For this review, use the dimensioned drawing (mm, ordinates from the lowest corner) and the shaded views. Coordinates: 2 decimals unless noted, no trailing zeros. Order: outer loops, then holes, each group sorted by start corner. A loop starts at its lowest first (then second) coordinate and runs counter-clockwise, first axis right, second up. Notation, with made-up numbers: (38, 89) -> (61, 89) arc R24 cw to (61, 103) -> close; hole circle Ø10 at (60, 37). An arc over 180 degrees is marked (long way). Return JSON: item names as keys, results as strings. Group by question number.
Item 1: Take a section at B-B (x = 43.1). Write out the cut boundary in (y, z), then the cut area to 3 significant figures.
Item 2: Take a section at A-A (z = 35.8). Write out the cut boundary in (x, y).
Item 3: Take a section at D-D (y = 2.15). Write out the cut boundary in (x, z).
Item 4: For line 1 along X through (y, z) = (2.3, 119.51); line 2 along X through (y, z) = (1.55, 5); line 3 along Z through (x, y) = (81, 1.35), list the stretches that pass through material, from the lowest coordinate up.
Item 5: Insertion check: pin 1 (1.5 mm diameter, centred on y = 2, z = 72.5, fed in from -X); pin 2 (0.9 mm diameter, centred on y = 1.5, z = 4.5, fed in from +X). Each pin has a flat end and moves straight along its axis. Give the tip position at first contact, or say it passes through.
Item 6: Take a section at C-C (z = 119.51). Write out the cut boundary in (x, y).
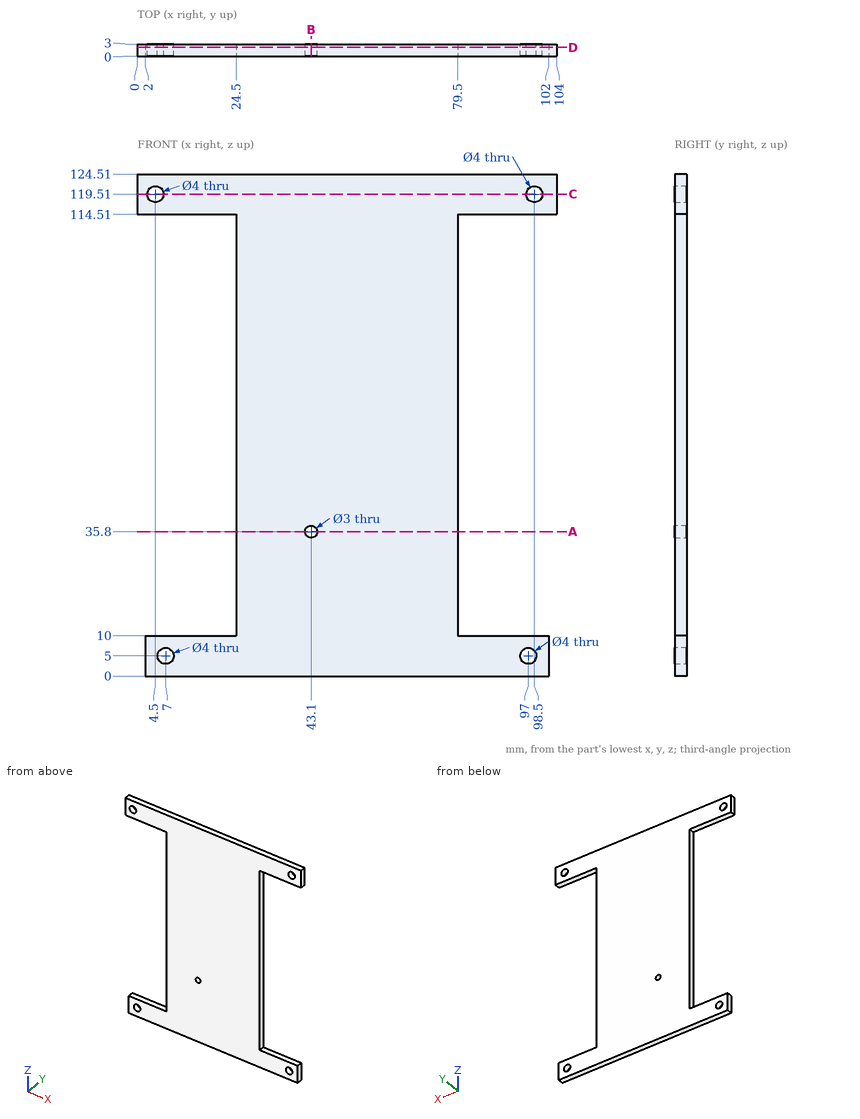
Findings below:
{
 "1": {"outline": "(0, 0) -> (3, 0) -> (3, 34.3) -> (0, 34.3) -> close; (0, 37.3) -> (3, 37.3) -> (3, 124.51) -> (0, 124.51) -> close", "area": "365 mm2"},
 "2": {"outline": "(24.5, 0) -> (41.6, 0) -> (41.6, 3) -> (24.5, 3) -> close; (44.6, 0) -> (79.5, 0) -> (79.5, 3) -> (44.6, 3) -> close"},
 "3": {"outline": "(0, 114.51) -> (24.5, 114.51) -> (24.5, 10) -> (2, 10) -> (2, 0) -> (102, 0) -> (102, 10) -> (79.5, 10) -> (79.5, 114.51) -> (104, 114.51) -> (104, 124.51) -> (0, 124.51) -> close; hole circle Ø4 at (4.5, 119.51); hole circle Ø4 at (7, 5); hole circle Ø3 at (43.1, 35.8); hole circle Ø4 at (97, 5); hole circle Ø4 at (98.5, 119.51)"},
 "4": {"line 1": "x = 0 to 2.5, 6.5 to 96.5, 100.5 to 104", "line 2": "x = 2 to 5, 9 to 95, 99 to 102", "line 3": "z = 0 to 10, 114.51 to 124.51"},
 "5": {"pin 1": "stops at x = 24.5", "pin 2": "stops at x = 102"},
 "6": {"outline": "(0, 0) -> (2.5, 0) -> (2.5, 3) -> (0, 3) -> close; (6.5, 0) -> (96.5, 0) -> (96.5, 3) -> (6.5, 3) -> close; (100.5, 0) -> (104, 0) -> (104, 3) -> (100.5, 3) -> close"}
}
